Can you work these out from the model? Positions are in its coordinate system, mm. A direction names the side the tool comes from. Coordinates: 2 decimals unless noted, no trailing zeros. Order: outer loops, then holes, each group sorted by start corner. A loop starts at its lowest first (then second) coordinate and runs counter-clockwise, first axis right, second up. Notation, with made-up numbers: (71, -33.5) -> (103, -33.5) arc R23 ccw to (103, -13.5) -> close; hole circle Ø5 at (6, 84.25). An arc over 180 degrees is marked (long way). Return JSON: item names as keys, results as strings. Group by question number.
1) Thinking about a two-plate mould opening in Y: for faces 1 (the flat face through (396.873, 49, 1376)), 2 (the flat face through (561, 30.05, 1375)), 3 (the cylindrical face through (391.94, 65.35, 1389.6)), which applies, +Y half, -Y half, draft (parallel to the pull), parting line (faces both ways), or undercut?
2) For pin 1 (6 mm diameter, centred on x = 563.5, z = 1377, fed in from +Y); pin 2 (24 mm diameter, centred on x = 502.5, z = 1372.5, fed in from +Y); pin 3 (0.8 mm diameter, centred on x = 586, z = 1383, fed in from +Y); pin 4 (4 mm diameter, centred on y = 34, z = 1390.46, fed in from -X), each with a flat end and sliding along its axis, tell me the tip position at first contact or that it passes through.
3) If I drill on probe 1 along X at (y, z) = (32, 1386); probe 2 along Z at (x, y) = (393.25, 64); probe 3 along X at (y, z) = (56.5, 1378.5), over which ranges is the centre line in solid material (lowest first)? Write a range as from..to.
4) If we section it at D-D, the plane x = 451.5: Please give me the cut outline in (y, z), then the cut area to 3 significant figures.
5) If we section it at B-B, the plane x = 561: Please give me the cut outline in (y, z).
6) If we section it at C-C, the plane y = 52.5: Please give me the cut outline in (x, z).
7) If we section it at A-A, the plane z = 1355.5: Please give me the cut outline in (x, y).
8) For faces 4 (the cylindrical face through (391.94, 64.07, 1361.56)), 5 (the cylindrical face through (391.94, 34.07, 1361.56)), 6 (the flat face through (386.873, 47, 1376)), 7 (the flat face through (413, 30, 1376)), 8 (the flat face through (555.358, 34, 1375)), which set-ups out of +Z, -Z, +X, -X, +Y, -Y let a thin tool reach every point of the face, with its end or its side?
from build123d import *

# Parameters (mm, degrees)
SKETCH1_W               = 226
SKETCH1_H               = 84
BOSS_EXTRUDE1_DEPTH     = 20
SKETCH9_W               = 215
SKETCH9_H               = 38.50000016
BOSS_EXTRUDE2_DEPTH     = 10
SKETCH12_W              = 10
SKETCH12_H              = 38.50000016
BOSS_EXTRUDE4_DEPTH     = 38
SKETCH14_R              = 1.6
CUT_EXTRUDE2_DEPTH      = 38
SKETCH18_W              = 173.6342166
SKETCH18_H              = 38.50000016
BOSS_EXTRUDE5_DEPTH     = 8
SKETCH20_W              = 226
SKETCH20_H              = 20
BOSS_EXTRUDE6_DEPTH     = 27.35
SKETCH20_4_W            = 226
SKETCH20_4_H            = 20
CUT_EXTRUDE3_DEPTH      = 27.35
SKETCH22_W              = 226
SKETCH22_H              = 20
CUT_EXTRUDE4_DEPTH      = 18.14670137
SKETCH23_W              = 38.50329863
SKETCH23_H              = 20
CUT_EXTRUDE5_DEPTH      = 11
SKETCH24_W              = 215
SKETCH24_H              = 38.50329863
CUT_EXTRUDE6_DEPTH      = 27
SKETCH27_W              = 31.3657834
SKETCH27_H              = 3
BOSS_EXTRUDE8_DEPTH     = 4.5
SKETCH28_W              = 31.3657834
SKETCH28_H              = 3
BOSS_EXTRUDE9_DEPTH     = 4.5
CUT_EXTRUDE9_DEPTH      = 5
CUT_EXTRUDE9_DEPTH_BACK = 14
SKETCH30_W              = 47.50000016
SKETCH30_H              = 11
CAVITY2_START           = 555.357736953
CAVITY2_DEPTH           = 12.45
CAVITY2_2_OUTLINE_W     = 9.75
CAVITY2_2_OUTLINE_H     = 10.05
CAVITY2_2_DEPTH         = 1.2
CAVITY2_START_2         = 566.607736953
CAVITY2_3_OUTLINE_W     = 9.75
CAVITY2_3_OUTLINE_H     = 10.05
CAVITY2_3_DEPTH         = 1.2
SKETCH32_W              = 10.05
SKETCH32_H              = 10.05
CUT_EXTRUDE14_DEPTH     = 10
SKETCH34_W              = 12.45
SKETCH34_H              = 12.45
BOSS_EXTRUDE11_DEPTH    = 3
SKETCH35_W              = 1.65
SKETCH35_H              = 46.5
CUT_EXTRUDE15_DEPTH     = 7


# Read off the part's stored shape, not the designer's step: Cavity2
with BuildPart() as part:
    # Sketch1 → Boss-Extrude1 (new body)
    with BuildSketch(Plane(origin=(375.872687737, 0, 1298.443562055), x_dir=(1, 0, 0), z_dir=(0, 1, 0))):
        with Locations((113, -81.370523073)):
            Rectangle(SKETCH1_W, SKETCH1_H)
    extrude(amount=BOSS_EXTRUDE1_DEPTH)

    # Sketch9 → Boss-Extrude2 (add)
    with BuildSketch(Plane(origin=(0, 20, 0), x_dir=(1, 0, 0), z_dir=(0, 1, 0))):
        with Locations((494.372687737, -1375.210786579)):
            Rectangle(SKETCH9_W, SKETCH9_H)
    extrude(amount=BOSS_EXTRUDE2_DEPTH)

    # Sketch12 → Boss-Extrude4 (add)
    with BuildSketch(Plane(origin=(0, 30, 0), x_dir=(1, 0, 0), z_dir=(0, 1, 0))):
        with Locations((391.872687737, -1375.210786579)):
            Rectangle(SKETCH12_W, SKETCH12_H)
    extrude(amount=BOSS_EXTRUDE4_DEPTH)

    # Sketch14 → Cut-Extrude2 (cut)
    with BuildSketch(Plane(origin=(396.872687737, 0, 0), x_dir=(0, 0, -1), z_dir=(1, 0, 0))):
        with Locations((-1390.460786659, 64)):
            Circle(SKETCH14_R)
        with Locations((-1359.960786499, 64)):
            Circle(SKETCH14_R)
        with Locations((-1390.460786659, 34)):
            Circle(SKETCH14_R)
        with Locations((-1359.960786499, 34)):
            Circle(SKETCH14_R)
    extrude(amount=-CUT_EXTRUDE2_DEPTH, mode=Mode.SUBTRACT)

    # Sketch18 → Boss-Extrude5 (add)
    with BuildSketch(Plane(origin=(0, 30, 0), x_dir=(1, 0, 0), z_dir=(0, 1, 0))):
        with Locations((515.055579437, -1375.210786579)):
            Rectangle(SKETCH18_W, SKETCH18_H)
    extrude(amount=BOSS_EXTRUDE5_DEPTH)

    # Sketch20 → Boss-Extrude6 (add)
    with BuildSketch(Plane.XY.offset(1421.814085128)):
        with Locations((488.872687737, 10)):
            Rectangle(SKETCH20_W, SKETCH20_H)
    extrude(amount=-BOSS_EXTRUDE6_DEPTH)

    # Sketch20<4> → Cut-Extrude3 (cut)
    with BuildSketch(Plane.XY.offset(1421.814085128)):
        with Locations((488.872687737, 10)):
            Rectangle(SKETCH20_4_W, SKETCH20_4_H)
    extrude(amount=-CUT_EXTRUDE3_DEPTH, mode=Mode.SUBTRACT)

    # Sketch22 → Cut-Extrude4 (cut)
    with BuildSketch(Plane(origin=(0, 0, 1337.814085128), x_dir=(-1, 0, 0), z_dir=(0, 0, -1))):
        with Locations((-488.872687737, 10)):
            Rectangle(SKETCH22_W, SKETCH22_H)
    extrude(amount=-CUT_EXTRUDE4_DEPTH, mode=Mode.SUBTRACT)

    # Sketch23 → Cut-Extrude5 (cut)
    with BuildSketch(Plane.ZY.offset(-375.872687737)):
        with Locations((1375.212435813, 10)):
            Rectangle(SKETCH23_W, SKETCH23_H)
    extrude(amount=-CUT_EXTRUDE5_DEPTH, mode=Mode.SUBTRACT)

    # Sketch24 → Cut-Extrude6 (cut)
    with BuildSketch(Plane.XZ):
        with Locations((494.372687737, 1375.212435813)):
            Rectangle(SKETCH24_W, SKETCH24_H)
    extrude(amount=-CUT_EXTRUDE6_DEPTH, mode=Mode.SUBTRACT)

    # Sketch27 → Boss-Extrude8 (add)
    with BuildSketch(Plane.XY.offset(1394.460786659)):
        Polygon((396.872687737, 68), (386.872687737, 68), (386.872687737, 27), (396.872687737, 27), (396.872687737, 30), align=None)
        with Locations((412.555579437, 28.5)):
            Rectangle(SKETCH27_W, SKETCH27_H)
        Polygon((428.238471137, 38), (428.238471137, 30), (428.238471137, 27), (601.872687737, 27), (601.872687737, 38), align=None)
    extrude(amount=BOSS_EXTRUDE8_DEPTH)

    # Sketch28 → Boss-Extrude9 (add)
    with BuildSketch(Plane(origin=(0, 0, 1355.960786499), x_dir=(-1, 0, 0), z_dir=(0, 0, -1))):
        Polygon((-428.238471137, 38), (-601.872687737, 38), (-601.872687737, 27), (-428.238471137, 27), (-428.238471137, 30), align=None)
        with Locations((-412.555579437, 28.5)):
            Rectangle(SKETCH28_W, SKETCH28_H)
        Polygon((-396.872687737, 68), (-396.872687737, 30), (-396.872687737, 27), (-386.872687737, 27), (-386.872687737, 68), align=None)
    extrude(amount=BOSS_EXTRUDE9_DEPTH)

    # Sketch30 → Cut-Extrude9 (cut, two sides: drawn at the far end of the back side and taken through both)
    with BuildSketch(Plane(origin=(601.872687737, 0, 0), x_dir=(0, 0, -1), z_dir=(1, 0, 0)).offset(-CUT_EXTRUDE9_DEPTH_BACK)):
        with Locations((-1375.210786579, 32.5)):
            Rectangle(SKETCH30_W, SKETCH30_H)
    extrude(amount=CUT_EXTRUDE9_DEPTH + CUT_EXTRUDE9_DEPTH_BACK, mode=Mode.SUBTRACT)

    # Cavity2 outline → Cavity2 (cut)
    with BuildSketch(Plane.YZ.offset(CAVITY2_START)):
        Polygon((27.05, 1368.985786659), (38, 1368.985786659), (38, 1370.185786659), (28.25, 1370.185786659), (28.25, 1380.235786659), (38, 1380.235786659), (38, 1381.435786659), (27.05, 1381.435786659), align=None)
    extrude(amount=CAVITY2_DEPTH, mode=Mode.SUBTRACT)

    # Cavity2 2 outline → Cavity2 2 (cut)
    with BuildSketch(Plane.YZ.offset(CAVITY2_START)):
        with Locations((33.125, 1375.210786659)):
            Rectangle(CAVITY2_2_OUTLINE_W, CAVITY2_2_OUTLINE_H)
    extrude(amount=CAVITY2_2_DEPTH, mode=Mode.SUBTRACT)

    # Cavity2 3 outline → Cavity2 3 (cut)
    with BuildSketch(Plane.YZ.offset(CAVITY2_START_2)):
        with Locations((33.125, 1375.210786659)):
            Rectangle(CAVITY2_3_OUTLINE_W, CAVITY2_3_OUTLINE_H)
    extrude(amount=CAVITY2_3_DEPTH, mode=Mode.SUBTRACT)

    # Cavity2 4 outline → Cavity2 4 (revolve, cut)
    with BuildSketch(Plane(origin=(0, 49.25, 1375.210786659), x_dir=(0, 1, 0), z_dir=(0, 0, -1))):
        Polygon((14.05, 428.238471137), (14.05, 454.238471137), (11.893245894, 454.238471137), (12.500000005, 454.857736959), (12.5, 553.357736953), (11.25, 553.357736953), (11.25, 428.238471137), align=None)
    revolve(axis=Axis((0, 49.25, 1375.210786659), (1, 0, 0)), mode=Mode.SUBTRACT)

    # Sketch32 → Cut-Extrude14 (cut)
    with BuildSketch(Plane(origin=(0, 38, 0), x_dir=(1, 0, 0), z_dir=(0, 1, 0))):
        with Locations((561.582736953, -1375.210786659)):
            Rectangle(SKETCH32_W, SKETCH32_H)
    extrude(amount=-CUT_EXTRUDE14_DEPTH, mode=Mode.SUBTRACT)

    # Sketch34 → Boss-Extrude11 (add)
    with BuildSketch(Plane(origin=(0, 27.05, 0), x_dir=(1, 0, 0), z_dir=(0, 1, 0))):
        with Locations((561.582736953, -1375.210786659)):
            Rectangle(SKETCH34_W, SKETCH34_H)
    extrude(amount=BOSS_EXTRUDE11_DEPTH)

    # Sketch35 → Cut-Extrude15 (cut)
    with BuildSketch(Plane(origin=(0, 38, 0), x_dir=(1, 0, 0), z_dir=(0, 1, 0))):
        with Locations((585.632736953, -1375.210786659)):
            Rectangle(SKETCH35_W, SKETCH35_H)
    extrude(amount=-CUT_EXTRUDE15_DEPTH, mode=Mode.SUBTRACT)


solid = part.part
Result sheet:
{
 "1": {"face 1": "draft", "face 2": "+Y half", "face 3": "undercut"},
 "2": {"pin 1": "stops at y = 30.05", "pin 2": "stops at y = 38", "pin 3": "stops at y = 31", "pin 4": "stops at x = 386.87"},
 "3": {"probe 1": "x = 386.87..396.87, 428.24..584.81, 586.46..587.87", "probe 2": "z = 1351.46..1358.36, 1361.56..1388.86, 1392.06..1398.96", "probe 3": "x = 386.87..396.87"},
 "4": {"outline": "(27, 1351.46) -> (38, 1351.46) -> (38, 1366.79) arc R14.05 cw to (38, 1383.63) -> (38, 1398.96) -> (27, 1398.96) -> close", "area": "490 mm2"},
 "5": {"outline": "(27, 1351.46) -> (38, 1351.46) -> (38, 1368.99) -> (30.05, 1368.99) -> (30.05, 1381.44) -> (38, 1381.44) -> (38, 1398.96) -> (27, 1398.96) -> close"},
 "6": {"outline": "(386.87, 1351.46) -> (396.87, 1351.46) -> (396.87, 1398.96) -> (386.87, 1398.96) -> close"},
 "7": {"outline": "(386.87, 27) -> (587.87, 27) -> (587.87, 38) -> (586.46, 38) -> (586.46, 31) -> (584.81, 31) -> (584.81, 38) -> (428.24, 38) -> (428.24, 30) -> (396.87, 30) -> (396.87, 68) -> (386.87, 68) -> close"},
 "8": {"face 4": "+X, -X", "face 5": "-X", "face 6": "+Z, -Z, -X, +Y, -Y", "face 7": "+Z, -Z, +Y", "face 8": "+Y"}
}
